```python
from build123d import *

# Parameters (mm, degrees)
F1_DEPTH = 2
F2_DEPTH = 15
F3_SIZE  = 1


with BuildPart() as f1:
    # F0 (on Top) → F1 (new body)
    with BuildSketch(Plane.XY):
        with BuildLine():
            Line((5, -10), (75, -10))
            ThreePointArc((75, -10), (85.606602, -5.606602), (90, 5))
            Line((90, 5), (90, 115))
            ThreePointArc((90, 115), (85.606602, 125.606602), (75, 130))
            Line((75, 130), (5, 130))
            ThreePointArc((5, 130), (-5.606602, 125.606602), (-10, 115))
            Line((-10, 115), (-10, 5))
            ThreePointArc((-10, 5), (-5.606602, -5.606602), (5, -10))
        make_face()
        with BuildLine():
            Line((75, 0), (5, 0))
            ThreePointArc((5, 0), (1.464466, 1.464466), (0, 5))
            Line((0, 5), (0, 115))
            ThreePointArc((0, 115), (1.464466, 118.535534), (5, 120))
            Line((5, 120), (75, 120))
            ThreePointArc((75, 120), (78.535534, 118.535534), (80, 115))
            Line((80, 115), (80, 5))
            ThreePointArc((80, 5), (78.535534, 1.464466), (75, 0))
        make_face(mode=Mode.SUBTRACT)
        with BuildLine():
            ThreePointArc((0, 5), (1.464466, 1.464466), (5, 0))
            Line((5, 0), (75, 0))
            ThreePointArc((75, 0), (78.535534, 1.464466), (80, 5))
            Line((80, 5), (80, 115))
            ThreePointArc((80, 115), (78.535534, 118.535534), (75, 120))
            Line((75, 120), (5, 120))
            ThreePointArc((5, 120), (1.464466, 118.535534), (0, 115))
            Line((0, 115), (0, 5))
        make_face()
        with BuildLine():
            Line((77, 114), (77, 6))
            ThreePointArc((77, 6), (76.12132, 3.87868), (74, 3))
            Line((74, 3), (6, 3))
            ThreePointArc((6, 3), (3.87868, 3.87868), (3, 6))
            Line((3, 6), (3, 114))
            ThreePointArc((3, 114), (3.87868, 116.12132), (6, 117))
            Line((6, 117), (74, 117))
            ThreePointArc((74, 117), (76.12132, 116.12132), (77, 114))
        make_face(mode=Mode.SUBTRACT)
    extrude(amount=F1_DEPTH)

    # F0 (on Top) → F2 (join)
    with BuildSketch(Plane.XY):
        with BuildLine():
            ThreePointArc((0, 5), (1.464466, 1.464466), (5, 0))
            Line((5, 0), (75, 0))
            ThreePointArc((75, 0), (78.535534, 1.464466), (80, 5))
            Line((80, 5), (80, 115))
            ThreePointArc((80, 115), (78.535534, 118.535534), (75, 120))
            Line((75, 120), (5, 120))
            ThreePointArc((5, 120), (1.464466, 118.535534), (0, 115))
            Line((0, 115), (0, 5))
        make_face()
        with BuildLine():
            Line((77, 114), (77, 6))
            ThreePointArc((77, 6), (76.12132, 3.87868), (74, 3))
            Line((74, 3), (6, 3))
            ThreePointArc((6, 3), (3.87868, 3.87868), (3, 6))
            Line((3, 6), (3, 114))
            ThreePointArc((3, 114), (3.87868, 116.12132), (6, 117))
            Line((6, 117), (74, 117))
            ThreePointArc((74, 117), (76.12132, 116.12132), (77, 114))
        make_face(mode=Mode.SUBTRACT)
    extrude(amount=-F2_DEPTH)

    # F3
    f3_edges = [f1.edges().sort_by_distance(p)[0] for p in [
        (77, 60, 2),
        (76.12132, 116.12132, 2),
        (40, 117, 2),
        (3.87868, 116.12132, 2),
        (3, 60, 2),
        (40, 3, 2),
        (76.12132, 3.87868, 2),
        (3.87868, 3.87868, 2),
        (-5.606602, -5.606602, 2),
        (40, -10, 2),
        (85.606602, -5.606602, 2),
        (90, 60, 2),
        (-10, 60, 2),
        (40, 130, 2),
        (-5.606602, 125.606602, 2),
        (85.606602, 125.606602, 2),
    ]]
    chamfer(f3_edges, length=F3_SIZE)


solid = f1.part
```
Geometry check sheet. Reference: the model listing, model coordinates, mm. A direction names the side the tool comes from. Round coordinates to 2 decimals unless told otherwise and drop trailing zeros. Loops run counter-clockwise (first coordinate to the right, second up) from the corner with the lowest first, then second, coordinate; pieces in that order, holes last. Notation, with made-up numbers: (66.25, 26) -> (90.25, 26) arc R26 ccw to (90.25, 62) -> close; hole circle Ø1 at (22, 50). An arc over 180 degrees is marked (long way). Use a Markdown table: item, result.
(1) Go/stop test with flat-tipped pins: P1, Ø4.5, axis at x = 26, z = -8, coming from the +Y side; P2, Ø2, axis at y = 8.5, z = -9, coming from the -X side; P3, Ø8, axis at x = 35, z = -4.5, coming from the -Y side. Record where each tip stops, or that it passes through.
Calculated:
| item | result |
|---|---|
| P1 | y = 120 |
| P2 | x = 0 |
| P3 | y = 0 |
(2) Scan lines: probe 1 along Y at (x, z) = (20, -13.75); probe 2 along X at (y, z) = (89.5, -8.25); probe 3 along Y at (x, z) = (18.5, 0.5). Record each from-to range of solid material in increasing order.
Calculated:
| item | result |
|---|---|
| probe 1 | 0 to 3, 117 to 120 |
| probe 2 | 0 to 3, 77 to 80 |
| probe 3 | -10 to 3, 117 to 130 |
(3) Sectioned sample at C-C (y = 61). Enter the section's corners in (x, z), then the cut area to 3 significant figures.
Calculated:
| item | result |
|---|---|
| outline | (-10, 0) -> (0, 0) -> (0, -15) -> (3, -15) -> (3, 1) -> (2, 2) -> (-9, 2) -> (-10, 1) -> close; (77, -15) -> (80, -15) -> (80, 0) -> (90, 0) -> (90, 1) -> (89, 2) -> (78, 2) -> (77, 1) -> close |
| area | 140 mm² |
(4) Sectioned sample at A-A (x = 55). Enter the section's corners in (y, z), then the cut area to 3 significant figures.
Calculated:
| item | result |
|---|---|
| outline | (-10, 0) -> (0, 0) -> (0, -15) -> (3, -15) -> (3, 1) -> (2, 2) -> (-9, 2) -> (-10, 1) -> close; (117, -15) -> (120, -15) -> (120, 0) -> (130, 0) -> (130, 1) -> (129, 2) -> (118, 2) -> (117, 1) -> close |
| area | 140 mm² |
(5) Sectioned sample at B-B (z = -5.25). Enter the section's corners in (x, y).
Calculated:
| item | result |
|---|---|
| outline | (0, 5) arc R5 ccw to (5, 0) -> (75, 0) arc R5 ccw to (80, 5) -> (80, 115) arc R5 ccw to (75, 120) -> (5, 120) arc R5 ccw to (0, 115) -> close; hole (3, 6) arc R3 ccw to (6, 3) -> (74, 3) arc R3 ccw to (77, 6) -> (77, 114) arc R3 ccw to (74, 117) -> (6, 117) arc R3 ccw to (3, 114) -> close |
(6) Set-up check for faces 1 (the flat face through (84, 61, 0)), 2 (the cylindrical face through (3.9, 3.86, -6.89)), 3 (the conical face through (3.652, 116.297, 1.285)), 4 (the cylindrical face through (79, 118, -7)): record each of +Z, -Z, +X, -X, +Y, -Y from which the full face is reachable in a straight line by a thin tool's end or side.
Calculated:
| item | result |
|---|---|
| face 1 | -Z |
| face 2 | +Z, -Z |
| face 3 | +Z |
| face 4 | -Z, +X, +Y |
(7) Mould release check, pull along Y, two halves, no side actions. Record for faces 5 (the conical face through (76.297, 116.348, 1.285)), 6 (the conical face through (-5.13, -4.91, 1.83)), 7 (the flat face through (0, 61, -7)): released by +Y, released by -Y, zero draft, split by the parting line, or undercut.
Calculated:
| item | result |
|---|---|
| face 5 | undercut |
| face 6 | released by -Y |
| face 7 | zero draft |
